Could you check a few things on this drawing? It's one solid part, dimensions in mm from its lowest x, y, z. Coordinates: 2 decimals unless noted, no trailing zeros. Loops run counter-clockwise (first coordinate to the right, second up) from the corner with the lowest first, then second, coordinate; pieces in that order, holes last.
1) Imagine slicing it at A-A on z = 25. Please give me the cut outline in (x, y), plus the area to 4 significant figures.
2) Imagine slicing it at B-B on x = 25. Please give me the cut outline in (y, z).
3) Imagine slicing it at C-C on y = 2.5. Please give me the cut outline in (x, z).
4) Will this pin go through, and if not, where does the flat tip stop? P1, Ø16, axis at x = 245, z = 15, coming from the +Y side.
5) If I drill on line 1 along X through (y, z) = (5, 19.5); line 2 along Z through (x, y) = (220, 2.75); line 3 along X through (y, z) = (6.25, 30.5), over which ranges is the centre line in solid material (lowest first)?
6) Imagine slicing it at D-D on z = 15. Please give me the cut outline in (x, y), plus the area to 3 significant figures.
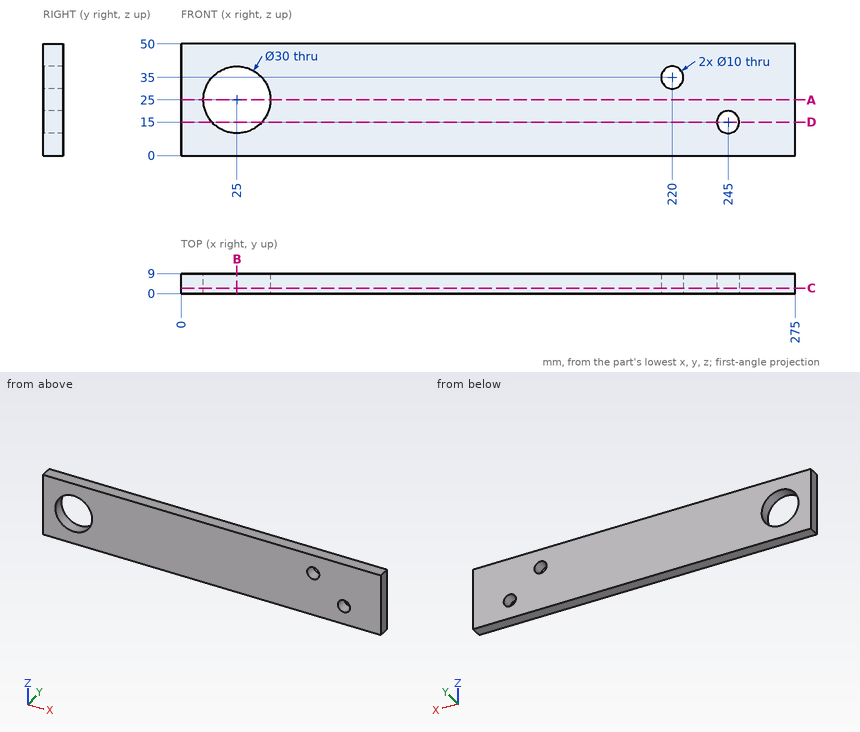
Filled in:
1. outline: (0, 0) - (10, 0) - (10, 9) - (0, 9) - close; (40, 0) - (275, 0) - (275, 9) - (40, 9) - close
1. area: 2,205 mm2
2. outline: (0, 0) - (9, 0) - (9, 10) - (0, 10) - close; (0, 40) - (9, 40) - (9, 50) - (0, 50) - close
3. outline: (0, 0) - (275, 0) - (275, 50) - (0, 50) - close; hole circle Ø30 at (25, 25); hole circle Ø10 at (220, 35); hole circle Ø10 at (245, 15)
4. P1: stops at y = 9
5. line 1: x = 0 to 11.04, 38.96 to 242.82, 247.18 to 275
5. line 2: z = 0 to 30, 40 to 50
5. line 3: x = 0 to 11.04, 38.96 to 217.82, 222.18 to 275
6. outline: (0, 0) - (13.82, 0) - (13.82, 9) - (0, 9) - close; (36.18, 0) - (240, 0) - (240, 9) - (36.18, 9) - close; (250, 0) - (275, 0) - (275, 9) - (250, 9) - close
6. area: 2,180 mm2
